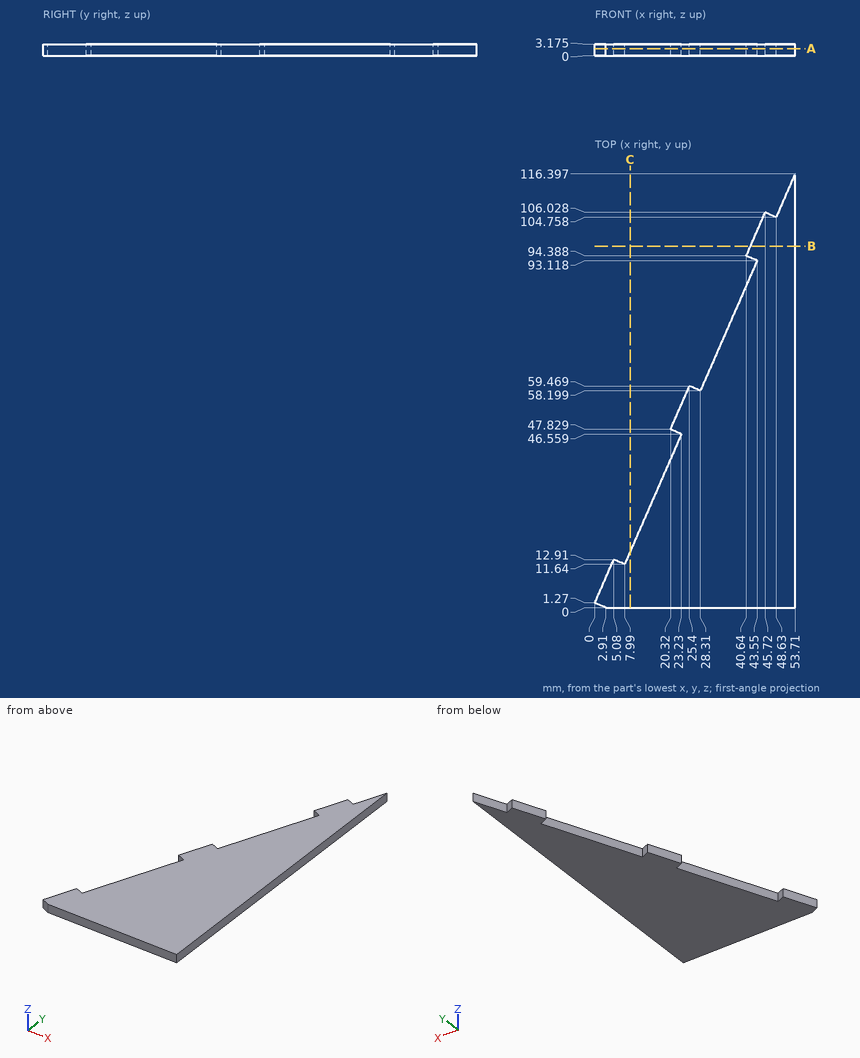
Geometry check sheet. Reference: drawing and pictorial views, mm from the part's lowest x, y, z. Round coordinates to 2 decimals unless told otherwise and drop trailing zeros. Loops run counter-clockwise (first coordinate to the right, second up) from the corner with the lowest first, then second, coordinate; pieces in that order, holes last. Notation, with made-up numbers: (55.25, -33) -> (90.25, -33) arc R12 cw to (90.25, -23) -> close; hole circle Ø9 at (19, 1). An arc over 180 degrees is marked (long way). Use a Markdown table: item, result.
(1) Sectioned sample at C-C (x = 9.5). Enter the section's corners in (y, z) (1 decimal).
Calculated:
| item | result |
|---|---|
| outline | (0, 0) -> (15.1, 0) -> (15.1, 3.2) -> (0, 3.2) -> close |
(2) Sectioned sample at B-B (y = 97). Enter the section's corners in (x, z) (1 decimal), then the cut area to 3 significant figures.
Calculated:
| item | result |
|---|---|
| outline | (41.8, 0) -> (53.7, 0) -> (53.7, 3.2) -> (41.8, 3.2) -> close |
| area | 37.9 mm² |
(3) Sectioned sample at A-A (z = 1.9). Enter the section's corners in (x, y), then the cut area to 3 significant figures.
Calculated:
| item | result |
|---|---|
| outline | (0, 1.27) -> (2.91, 0) -> (53.71, 0) -> (53.71, 116.4) -> (48.63, 104.76) -> (45.72, 106.03) -> (40.64, 94.39) -> (43.55, 93.12) -> (28.31, 58.2) -> (25.4, 59.47) -> (20.32, 47.83) -> (23.23, 46.56) -> (7.99, 11.64) -> (5.08, 12.91) -> close |
| area | 3,080 mm² |
(4) Scan lines: probe 1 along X at (y, z) = (31, 1.75); probe 2 along Y at (x, z) = (20, 0.6) (1 decimal); probe 3 along Y at (x, z) = (13.5, 0.35) (1 decimal). Record each from-to range of solid material in increasing order.
Calculated:
| item | result |
|---|---|
| probe 1 | 16.44 to 53.71 |
| probe 2 | 0 to 39.2 |
| probe 3 | 0 to 24.3 |
